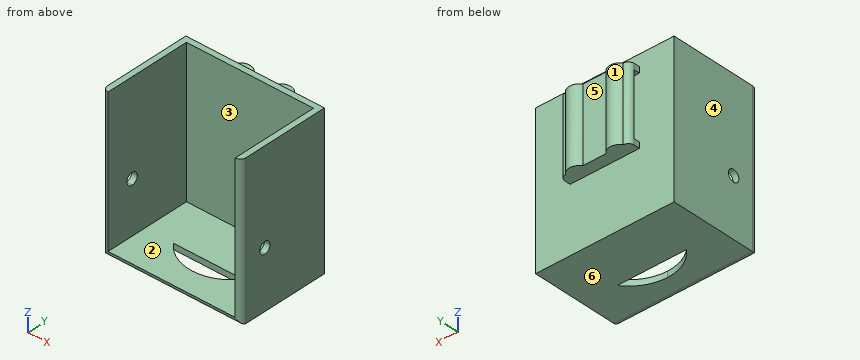
from build123d import *

# Parameters (mm, degrees)
F1_DEPTH      = 5
F2_DEPTH      = 125
F4_DEPTH      = 25
F4_DEPTH_BACK = 129
F5_W          = 60
F5_H          = 5
F6_DEPTH      = 10
F7_W          = 60
F7_H          = 5
F8_DEPTH      = 54
F9_R          = 4.99999
F11_DEPTH     = 64


# Not quite as in the source:
# - a fillet or chamfer is up to 0.001 mm smaller than in the source, because OpenCascade refuses the exact size
# - ends of sketch curves that miss each other by under 0.0002 mm in the source are joined


with BuildPart() as f1:
    # F0 (on Top) → F1 (new body)
    with BuildSketch(Plane.XY):
        Polygon((55, -40), (60, -40), (60, 40), (-60, 40), (-60, -40), (-55, -40), (-55, 35), (0, 35), (55, 35), align=None)
        with BuildLine():
            Line((-55, -40), (0, -40))
            Line((0, -40), (0, -20))
            ThreePointArc((0, -20), (-16.7705098312, -16.0410196625), (-30, -5))
            Line((-30, -5), (0, -5))
            Line((0, -5), (0, 35))
            Line((0, 35), (-55, 35))
            Line((-55, 35), (-55, -40))
        make_face()
        with BuildLine():
            Line((0, -40), (55, -40))
            Line((55, -40), (55, 35))
            Line((55, 35), (0, 35))
            Line((0, 35), (0, -5))
            Line((0, -5), (30, -5))
            ThreePointArc((30, -5), (16.7705098312, -16.0410196625), (0, -20))
            Line((0, -20), (0, -40))
        make_face()
    extrude(amount=-F1_DEPTH)

    # F0 (on Top) → F2 (join)
    with BuildSketch(Plane.XY):
        Polygon((55, -40), (60, -40), (60, 40), (-60, 40), (-60, -40), (-55, -40), (-55, 35), (0, 35), (55, 35), align=None)
    extrude(amount=F2_DEPTH)

    # F3 (on face) → F4 (cut, two sides)
    with BuildSketch(Plane.YZ.offset(-55)) as f4_sk:
        with BuildLine():
            Line((-17, 45), (-17, 40))
            ThreePointArc((-17, 40), (-13.4644660941, 41.4644660941), (-12, 45))
            Line((-12, 45), (-17, 45))
        make_face()
        with BuildLine():
            ThreePointArc((-12, 45), (-20.5355339059, 48.5355339059), (-17, 40))
            Line((-17, 40), (-17, 45))
            Line((-17, 45), (-12, 45))
        make_face()
    extrude(amount=-F4_DEPTH, mode=Mode.SUBTRACT)
    extrude(f4_sk.sketch, amount=F4_DEPTH_BACK, mode=Mode.SUBTRACT)

    # F5 (on face) → F6 (join)
    with BuildSketch(Plane(origin=(0, 40, 0), x_dir=(-1, 0, 0), z_dir=(0, 1, 0))):
        Polygon((30, 115), (0, 115), (-30, 115), (-30, 110), (30, 110), align=None)
        with Locations((0, 53.5)):
            Rectangle(F5_W, F5_H)
    extrude(amount=F6_DEPTH)

    # F7 (on face) → F8 (join, through all)
    with BuildSketch(Plane(origin=(0, 0, 110), x_dir=(1, 0, 0), z_dir=(0, 0, -1))):
        with Locations((0, -47.5)):
            Rectangle(F7_W, F7_H)
    extrude(amount=F8_DEPTH)

    # F9 (radius 5 in the source; OpenCascade refuses exactly that, so slightly less here)
    f9_edges = [f1.edges().sort_by_distance(p)[0] for p in [
        (-60, -40, 60),
        (0, -40, -5),
        (60, -40, 60),
        (-30, 50, 83),
        (30, 50, 83),
    ]]
    fillet(f9_edges, radius=F9_R)

    # F10 (on face) → F11 (join, through all)
    with BuildSketch(Plane.XY.offset(115)):
        with BuildLine():
            ThreePointArc((-17.5, 54), (-21.75, 52.9375), (-25, 50))
            Line((-25, 50), (-17.5, 50))
            Line((-17.5, 50), (-17.5, 54))
        make_face()
        with BuildLine():
            Line((-17.5, 54), (-17.5, 50))
            Line((-17.5, 50), (-10, 50))
            ThreePointArc((-10, 50), (-13.25, 52.9375), (-17.5, 54))
        make_face()
        with BuildLine():
            ThreePointArc((25, 50), (17.5, 54), (10, 50))
            Line((10, 50), (25, 50))
        make_face()
    extrude(amount=-F11_DEPTH)


solid = f1.part
Input: part model. Units: mm. Frame: model coordinates. Face numbers are marked on the shaded views. A direction names the side the tool comes from. Give positions to 0.01 mm unless a question says otherwise; leave off trailing zeros. Write each loop counter-clockwise with the first axis right and the second up, starting at its lowest first coordinate (ties: lowest second). Pieces come first, ordered by that corner, then holes.
Q1. Set-up query: the marked faces 1 and 2. Return all of +Z, -Z, +X, -X, +Y, -Y with unobstructed straight access to the full face (end or side cutting, diameter ignored); none if empty.
Q2. Section A-A, the plane x = -2. State how many separate pieces and enclosed holes the cut face has, plus the area to 3 significant figures.
Q3. Pull-direction query (X, two-part tool) for the marked faces 3, 4, 5 and 6; classes: pulls with the +X half, pulls with the -X half, needs draft (parallel to the pull), parting line crosses it, or undercut.
Q4. First-contact query: P1, Ø2.5, axis at y = 42, z = 87.5, coming from the +X side; P2, Ø4, axis at x = 45, y = -30.5, coming from the +Z side; P3, Ø4, axis at x = 13.5, y = 45.5, coming from the -Z side; P4, Ø1, axis at x = -33, z = 19.5, coming from the +Y side. Flat tips, straight axial feed; report the tip coordinate or a pass-through.
Q5. Section C-C, the plane y = -2. Output: boundary loops of the cut face in (x, z), plus the area to 3 significant figures.
Q6. Material intervals for probe 1 along Z at (x, y) = (-58, -17); probe 2 along X at (y, z) = (8.5, 5.5); probe 3 along Y at (x, z) = (-1, 106), sorted ascending.
Filled in:
1. face 1: +Z, -Z, +Y
1. face 2: +Z, -Y
2. separate pieces: 2
2. enclosed holes: 1
2. area: 1,310 mm2
3. face 3: undercut
3. face 4: pulls with the -X half
3. face 5: undercut
3. face 6: needs draft
4. P1: passes through
4. P2: stops at z = 0
4. P3: stops at z = 51
4. P4: stops at y = 40
5. outline: (-60, -5) - (60, -5) - (60, 125) - (55, 125) - (55, 0) - (-55, 0) - (-55, 125) - (-60, 125) - close
5. area: 1,850 mm2
6. probe 1: z = -5 to 40, 50 to 125
6. probe 2: x = -60 to -55, 55 to 60
6. probe 3: y = 35 to 40, 45 to 50
